Read the model definition and answer for the solid it produces. Units are mm, in the model's axes. A direction names the side the tool comes from. Coordinates: 2 decimals unless noted, no trailing zeros. Write each loop counter-clockwise with the first axis right and the second up, starting at its lowest first coordinate (ties: lowest second). Pieces come first, ordered by that corner, then holes. Notation, with made-up numbers: (36, 14) - (92, 14) arc R16 cw to (92, 22) - close; hole circle Ø10 at (-6, 60). An arc over 180 degrees is marked (long way). Use a Markdown table: item, result.
from build123d import *

# Parameters (mm, degrees)
ESQUISSE1_R        = 21
BOSS_EXTRU_1_DEPTH = 22
BOSS_EXTRU_2_DEPTH = 10
ESQUISSE3_R        = 20
BOSS_EXTRU_3_DEPTH = 3.2
ESQUISSE4_R        = 21
BOSS_EXTRU_4_DEPTH = 43.2
ESQUISSE5_R        = 14
BOSS_EXTRU_5_DEPTH = 2.8
ESQUISSE6_R        = 7.75
BOSS_EXTRU_6_DEPTH = 1.9
ESQUISSE7_R        = 6
BOSS_EXTRU_7_DEPTH = 7.8
BOSS_EXTRU_8_DEPTH = 10.5


with BuildPart() as part:
    # Esquisse1 → Boss.-Extru.1 (new body)
    with BuildSketch(Plane.XY):
        Circle(ESQUISSE1_R)
    extrude(amount=BOSS_EXTRU_1_DEPTH)

    # Esquisse2 → Boss.-Extru.2 (add)
    with BuildSketch(Plane(origin=(0, 0, 0), x_dir=(-1, 0, 0), z_dir=(0, 0, -1))):
        with BuildLine():
            ThreePointArc((9.15, -18.90178563), (0, -21), (-9.15, -18.90178563))
            Line((-9.15, -18.90178563), (-9.15, -26))
            Line((-9.15, -26), (9.15, -26))
            Line((9.15, -26), (9.15, -18.90178563))
        make_face()
    extrude(amount=-BOSS_EXTRU_2_DEPTH)

    # Esquisse3 → Boss.-Extru.3 (add)
    with BuildSketch(Plane.XY.offset(22)):
        Circle(ESQUISSE3_R)
    extrude(amount=BOSS_EXTRU_3_DEPTH)

    # Esquisse4 → Boss.-Extru.4 (add)
    with BuildSketch(Plane.XY.offset(25.2)):
        Circle(ESQUISSE4_R)
    extrude(amount=BOSS_EXTRU_4_DEPTH)

    # Esquisse5 → Boss.-Extru.5 (add)
    with BuildSketch(Plane.XY.offset(68.4)):
        Circle(ESQUISSE5_R)
    extrude(amount=BOSS_EXTRU_5_DEPTH)

    # Esquisse6 → Boss.-Extru.6 (add)
    with BuildSketch(Plane.XY.offset(71.2)):
        Circle(ESQUISSE6_R)
    extrude(amount=BOSS_EXTRU_6_DEPTH)

    # Esquisse7 → Boss.-Extru.7 (add)
    with BuildSketch(Plane.XY.offset(73.1)):
        Circle(ESQUISSE7_R)
    extrude(amount=BOSS_EXTRU_7_DEPTH)

    # Esquisse8 → Boss.-Extru.8 (add)
    with BuildSketch(Plane.XY.offset(80.9)):
        with BuildLine():
            ThreePointArc((6, 0), (2.449489743, 5.477225575), (-4, 4.472135955))
            Line((-4, 4.472135955), (-4, -4.472135955))
            ThreePointArc((-4, -4.472135955), (2.449489743, -5.477225575), (6, 0))
        make_face()
    extrude(amount=BOSS_EXTRU_8_DEPTH)


solid = part.part
(1) The mould has two halves that part along Z. Classify faces 1 (the flat face through (-4, 0, 86)), 2 (the flat face through (19, -8, 25.2)), 3 (the flat face through (1, 0, 91.4)): pulls with the +Z half, pulls with the -Z half, needs draft (parallel to the pull), parting line crosses it, or undercut.
Report:
| item | result |
|---|---|
| face 1 | needs draft |
| face 2 | undercut |
| face 3 | pulls with the +Z half |
(2) Straight lines are drawn through the part: L1, parallel to Z at x = 17, y = 11.5; L2, parallel to Z at x = -16, y = -11.5; L3, parallel to Z at x = -5.5, y = -1. For each, find the intervals that lie inside material, in ascending order.
Report:
| item | result |
|---|---|
| L1 | z = 0 to 22, 25.2 to 68.4 |
| L2 | z = 0 to 68.4 |
| L3 | z = 0 to 80.9 |
(3) A cutting plane is placed at B-B, the plane x = 0. Write down the section's boundary in (y, z), and give its area (3 significant figures).
Report:
| item | result |
|---|---|
| outline | (-26, 0) - (21, 0) - (21, 22) - (20, 22) - (20, 25.2) - (21, 25.2) - (21, 68.4) - (14, 68.4) - (14, 71.2) - (7.75, 71.2) - (7.75, 73.1) - (6, 73.1) - (6, 91.4) - (-6, 91.4) - (-6, 73.1) - (-7.75, 73.1) - (-7.75, 71.2) - (-14, 71.2) - (-14, 68.4) - (-21, 68.4) - (-21, 25.2) - (-20, 25.2) - (-20, 22) - (-21, 22) - (-21, 10) - (-26, 10) - close |
| area | 3,240 mm² |
(4) For faces 4 (the flat face through (-9.15, -23, 5)), 5 (the flat face through (9.15, -22, 5)), 6 (the cylindrical face through (-4.336, -19.524, 23.578)), 7 (the flat face through (6, -6, 71.2)), 8 (the flat face through (-5, 0, 80.9)), determine the directions among +Z, -Z, +X, -X, +Y, -Y from which every point of the face is accessible in a straight line to the end or side of a thin tool.
Report:
| item | result |
|---|---|
| face 4 | +Z, -Z, -X, -Y |
| face 5 | +Z, -Z, +X, -Y |
| face 6 | none |
| face 7 | +Z |
| face 8 | +Z, -X, +Y, -Y |
(5) A cutting plane is placed at A-A, the plane y = -17.5. Write down the section's boundary in (x, z).
Report:
| item | result |
|---|---|
| outline | (-11.61, 0) - (11.61, 0) - (11.61, 22) - (9.68, 22) - (9.68, 25.2) - (11.61, 25.2) - (11.61, 68.4) - (-11.61, 68.4) - (-11.61, 25.2) - (-9.68, 25.2) - (-9.68, 22) - (-11.61, 22) - close |
(6) Each of these flat-tipped pins is pushed along its axis until it touches: P1, Ø8, axis at y = 4.5, z = 16.5, coming from the +X side; P2, Ø5.5, axis at y = -22, z = 3, coming from the -X side; P3, Ø5, axis at y = -17, z = 14.5, coming from the -X side. Where does it stop, or does it pass through?
Report:
| item | result |
|---|---|
| P1 | stops at x = 20.99 |
| P2 | stops at x = -9.15 |
| P3 | stops at x = -15.19 |
(7) A cutting plane is placed at D-D, the plane x = 12.5. Write down the section's boundary in (y, z).
Report:
| item | result |
|---|---|
| outline | (-16.87, 0) - (16.87, 0) - (16.87, 22) - (15.61, 22) - (15.61, 25.2) - (16.87, 25.2) - (16.87, 68.4) - (6.3, 68.4) - (6.3, 71.2) - (-6.3, 71.2) - (-6.3, 68.4) - (-16.87, 68.4) - (-16.87, 25.2) - (-15.61, 25.2) - (-15.61, 22) - (-16.87, 22) - close |
(8) A cutting plane is placed at C-C, the plane z = 61. Write down the section's boundary in (x, y).
Report:
| item | result |
|---|---|
| outline | circle Ø42 at (0, 0) |
